Check sheet for the modelled part. Datum: model origin and axes. Units: mm. A direction names the side the tool comes from. Round coordinates to 2 decimals unless told otherwise and drop trailing zeros. Order: outer loops, then holes, each group sorted by start corner. A loop starts at its lowest first (then second) coordinate and runs counter-clockwise, first axis right, second up.
from build123d import *

# Parameters (mm, degrees)
SKETCH1_R           = 127
BOSS_EXTRUDE1_DEPTH = 12.7
SKETCH2_R           = 12.7
CUT_EXTRUDE1_DEPTH  = 12.7
SKETCH3_R           = 76.2
BOSS_EXTRUDE2_DEPTH = 254
BOSS_EXTRUDE3_START = 12.7
SKETCH4_R           = 127
BOSS_EXTRUDE3_DEPTH = 12.7
CUT_EXTRUDE2_START  = -12.7
SKETCH5_R           = 12.7
CUT_EXTRUDE2_DEPTH  = 12.7
FILLET1_R           = 12.7
SKETCH6_R           = 50.8
CUT_EXTRUDE3_DEPTH  = 325.12


with BuildPart() as part:
    # Sketch1 → Boss-Extrude1 (new body)
    with BuildSketch(Plane(origin=(0, 0, 0), x_dir=(1, 0, 0), z_dir=(0, 1, 0))):
        with Locations(Location((0, 0, 0), (0, 0, 270))):
            Circle(SKETCH1_R)
    extrude(amount=BOSS_EXTRUDE1_DEPTH)

    # Sketch2 → Cut-Extrude1 (cut)
    with BuildSketch(Plane(origin=(0, 12.7, 0), x_dir=(1, 0, 0), z_dir=(0, 1, 0))):
        with Locations(Location((0, 107.95, 0), (0, 0, 270))):
            Circle(SKETCH2_R)
        with Locations(Location((0, -107.95, 0), (0, 0, 270))):
            Circle(SKETCH2_R)
        with Locations(Location((-93.6625, 53.975, 0), (0, 0, 270))):
            Circle(SKETCH2_R)
        with Locations(Location((93.6625, 53.975, 0), (0, 0, 270))):
            Circle(SKETCH2_R)
        with Locations(Location((-93.6625, -53.975, 0), (0, 0, 270))):
            Circle(SKETCH2_R)
        with Locations(Location((93.6625, -53.975, 0), (0, 0, 270))):
            Circle(SKETCH2_R)
    extrude(amount=-CUT_EXTRUDE1_DEPTH, mode=Mode.SUBTRACT)

    # Sketch3 → Boss-Extrude2 (add)
    with BuildSketch(Plane.XZ):
        with Locations(Location((0, 0, 0), (0, 0, 90))):
            Circle(SKETCH3_R)
    extrude(amount=BOSS_EXTRUDE2_DEPTH)

    # Sketch4 → Boss-Extrude3 (add)
    with BuildSketch(Plane.XZ.offset(254).offset(BOSS_EXTRUDE3_START)):
        with Locations(Location((0, 0, 0), (0, 0, 90))):
            Circle(SKETCH4_R)
    extrude(amount=-BOSS_EXTRUDE3_DEPTH)

    # Sketch5 → Cut-Extrude2 (cut)
    with BuildSketch(Plane.XZ.offset(266.7).offset(CUT_EXTRUDE2_START)):
        with Locations(Location((0, 107.95, 0), (0, 0, 90))):
            Circle(SKETCH5_R)
        with Locations(Location((5.510274908, -107.95, 0), (0, 0, 270))):
            Circle(SKETCH5_R)
        with Locations(Location((-93.6625, 53.975, 0), (0, 0, 90))):
            Circle(SKETCH5_R)
        with Locations(Location((93.6625, 53.975, 0), (0, 0, 90))):
            Circle(SKETCH5_R)
        with Locations(Location((-93.6625, -53.975, 0), (0, 0, 90))):
            Circle(SKETCH5_R)
        with Locations(Location((93.6625, -53.975, 0), (0, 0, 90))):
            Circle(SKETCH5_R)
    extrude(amount=CUT_EXTRUDE2_DEPTH, mode=Mode.SUBTRACT)

    # Fillet1
    fillet1_edges = [part.edges().sort_by_distance(p)[0] for p in [
        (0, 0, -76.2),
        (0, -254, -76.2),
    ]]
    fillet(fillet1_edges, radius=FILLET1_R)

    # Sketch6 → Cut-Extrude3 (cut)
    with BuildSketch(Plane(origin=(0, 12.7, 0), x_dir=(1, 0, 0), z_dir=(0, 1, 0))):
        with Locations(Location((0, 0, 0), (0, 0, 270))):
            Circle(SKETCH6_R)
    extrude(amount=-CUT_EXTRUDE3_DEPTH, mode=Mode.SUBTRACT)


solid = part.part
1) Sectioned sample at D-D on x = 0. Count the separate pieces of the cut face and the enclosed holes in it, and give its area (3 significant figures).
2) Set-up check for faces 4 (the face through (-102.246, -260.261, -63.335)), 5 (the face through (-7.728, 6.439, -118.028)), 6 (the face through (-76, -254, -48)), 7 (the face through (6.069, -260.261, -95.262)): record each of +Z, -Z, +X, -X, +Y, -Y from which the full face is reachable in a straight line by a thin tool's end or side.
3) Scan lines: line 1 (Y direction, x = -87, z = -83); line 2 (X direction, y = -227.5, z = 0); line 3 (X direction, y = -3.5, z = 35). Record each from-to range of solid material in increasing order.
4) Gauge pin test, flat ends, axial feed: pin 1 (3 mm diameter, centred on y = -36.5, z = -60, fed in from +X); pin 2 (23 mm diameter, centred on x = 5.51, z = -107.95, fed in from -Y); pin 3 (1.5 mm diameter, centred on x = -51, y = -99, fed in from +Z). Record the tip position at first contact, or that the pin passes through.
5) Sectioned sample at C-C on y = -199. Record the cut outline in (x, z), and give its area (3 significant figures).
6) Sectioned sample at A-A on z = 0. Record the cut outline in (x, y).
7) Draft check along Z on faces 1 (the face through (85, 0, -38)), 2 (the face through (123.98, -260.44, -27.53)), 3 (the face through (85.079, -260.261, -63.335)). Enter one of: pulls with the +Z half, pulls with the -Z half, needs draft (parallel to the pull), parting line crosses it, or undercut.
8) Sectioned sample at B-B on z = 107.95. Record the cut outline in (x, y).
Values found:
1. separate pieces: 6
1. enclosed holes: 0
1. area: 15,700 mm2
2. face 4: +Y, -Y
2. face 5: +Y
2. face 6: none
2. face 7: -Y
3. line 1: y = -266.7 to -254, 0 to 12.7
3. line 2: x = -76.2 to -50.8, 50.8 to 76.2
3. line 3: x = -72.1 to -36.82, 36.82 to 72.1
4. pin 1: stops at x = 48.83
4. pin 2: stops at y = 0
4. pin 3: stops at z = 57.28
5. outline: circle Ø152.4 at (0, 0); hole circle Ø101.6 at (0, 0)
5. area: 10,100 mm2
6. outline: (-127, -266.7) - (-50.8, -266.7) - (-50.8, 12.7) - (-127, 12.7) - (-127, 0) - (-88.9, 0) arc R12.7 cw to (-76.2, -12.7) - (-76.2, -241.3) arc R12.7 cw to (-88.9, -254) - (-127, -254) - close; (50.8, -266.7) - (127, -266.7) - (127, -254) - (88.9, -254) arc R12.7 cw to (76.2, -241.3) - (76.2, -12.7) arc R12.7 cw to (88.9, 0) - (127, 0) - (127, 12.7) - (50.8, 12.7) - close
7. face 1: needs draft
7. face 2: parting line crosses it
7. face 3: undercut
8. outline: (-66.9, -266.7) - (-12.7, -266.7) - (-12.7, -254) - (-66.9, -254) - close; (-66.9, 0) - (-12.7, 0) - (-12.7, 12.7) - (-66.9, 12.7) - close; (12.7, -266.7) - (66.9, -266.7) - (66.9, -254) - (12.7, -254) - close; (12.7, 0) - (66.9, 0) - (66.9, 12.7) - (12.7, 12.7) - close
